Can you work these out from the drawing? Everything is in mm from the part's minimum corner. A direction names the side the tool comes from. Give positions to 0.01 mm unless a question says otherwise; leave off trailing zeros. Loops run counter-clockwise (first coordinate to the right, second up) from the corner with the lowest first, then second, coordinate; pieces in that order, holes last. Notation, with made-up numbers: (87.25, 30.25) - (124.25, 30.25) arc R29 cw to (124.25, 58.25) - close; hole circle Ø3 at (84, 34). An arc over 180 degrees is marked (long way). Answer in a Markdown table with one row per item.
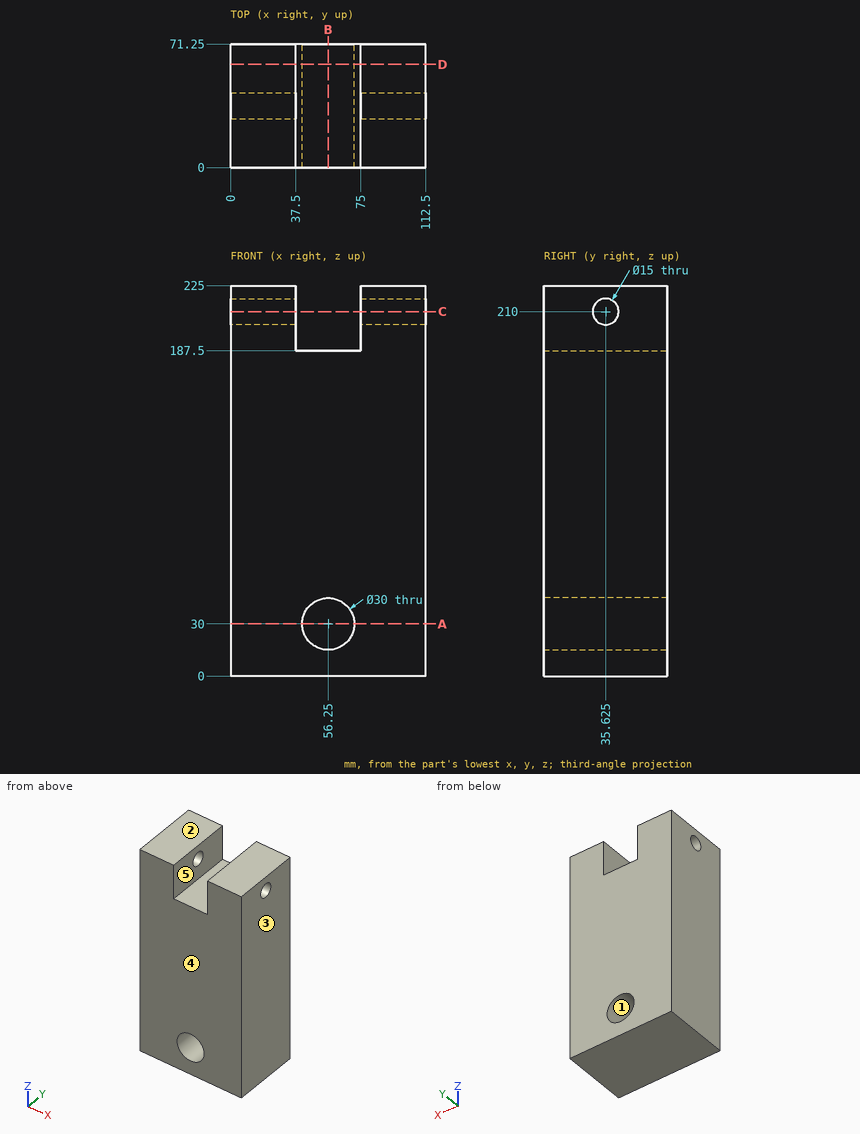
Q1. If I drill on line 1 (X direction, y = 20.5, z = 188); line 2 (X direction, y = 21, z = 30); line 3 (Y direction, x = 29.5, z = 210) (3 decimals), over which ranges is the centre line in solid material (lowest first)? Write a range as [from, to].
Checked values:
| item | result |
|---|---|
| line 1 | x = [0, 37.5], [75, 112.5] |
| line 2 | x = [0, 41.25], [71.25, 112.5] |
| line 3 | y = [0, 28.125], [43.125, 71.25] |
Q2. Imagine slicing it at C-C, the plane z = 210. Write out the boundary of the cut face in (x, y) (3 decimals), and give its area (3 significant figures).
Checked values:
| item | result |
|---|---|
| outline | (0, 0) - (37.5, 0) - (37.5, 28.125) - (0, 28.125) - close; (0, 43.125) - (37.5, 43.125) - (37.5, 71.25) - (0, 71.25) - close; (75, 0) - (112.5, 0) - (112.5, 28.125) - (75, 28.125) - close; (75, 43.125) - (112.5, 43.125) - (112.5, 71.25) - (75, 71.25) - close |
| area | 4,220 mm² |
Q3. Imagine slicing it at B-B, the plane x = 56.25. Write out the boundary of the cut face in (y, z), and give its area (3 significant figures).
Checked values:
| item | result |
|---|---|
| outline | (0, 0) - (71.25, 0) - (71.25, 15) - (0, 15) - close; (0, 45) - (71.25, 45) - (71.25, 187.5) - (0, 187.5) - close |
| area | 11,200 mm² |
Q4. Imagine slicing it at A-A, the plane z = 30. Write out the boundary of the cut face in (x, y).
Checked values:
| item | result |
|---|---|
| outline | (0, 0) - (41.25, 0) - (41.25, 71.25) - (0, 71.25) - close; (71.25, 0) - (112.5, 0) - (112.5, 71.25) - (71.25, 71.25) - close |
Q5. On a 3-axis mill with a long thin cutter (end or side, diameter ignored), from which of +Z, -Z, +X, -X, +Y, -Y can I reach the whole of each face in a straight line? I mean the marked faces 4 and 5. Say none if no direction works.
Checked values:
| item | result |
|---|---|
| face 4 | +Z, -Z, +X, -X, -Y |
| face 5 | +Z, +Y, -Y |
Q6. Imagine slicing it at D-D, the plane y = 59.5. Write out the boundary of the cut face in (x, z), and give its area (3 significant figures).
Checked values:
| item | result |
|---|---|
| outline | (0, 0) - (112.5, 0) - (112.5, 225) - (75, 225) - (75, 187.5) - (37.5, 187.5) - (37.5, 225) - (0, 225) - close; hole circle Ø30 at (56.25, 30) |
| area | 23,200 mm² |
Q7. If we mould it in two halves opening along Z, with no side actions, what happens to the marked faces 1, 2 and 3? For each: released by +Z, released by -Z, zero draft, split by the parting line, or undercut.
Checked values:
| item | result |
|---|---|
| face 1 | undercut |
| face 2 | released by +Z |
| face 3 | zero draft |
Q8. For pin 1 (11 mm diameter, centred on x = 65, y = 21.5, fed in from +Z), with a flat end and sliding along its axis, tell me the tip position at first contact or that it passes through.
Checked values:
| item | result |
|---|---|
| pin 1 | stops at z = 187.5 |
